from build123d import *

# Parameters (mm, degrees)
SKETCH2_R           = 31
SKETCH2_R_2         = 11.1
SKETCH2_R_3         = 3
BOSS_EXTRUDE1_DEPTH = 6
BOSS_EXTRUDE3_START = -3.9
SKETCH4_R           = 11.1
SKETCH4_R_2         = 5
BOSS_EXTRUDE3_DEPTH = 3.9
SKETCH5_R           = 2.3
CUT_EXTRUDE1_DEPTH  = 6
CIRPATTERN3_COUNT   = 4
CUT_EXTRUDE2_REACH  = 101.674
SKETCH12_R          = 3
CIRPATTERN4_COUNT   = 2
CIRPATTERN4_ANGLE   = 60
CIRPATTERN5_COUNT   = 4


# Read off the part's stored shape, not the designer's step: Revolve1
with BuildPart() as part:
    # Sketch2 → Boss-Extrude1 (new body)
    with BuildSketch(Plane(origin=(-62.154924708, 3.943558292, 10.8), x_dir=(1, 0, 0), z_dir=(0, 0, 1))):
        Circle(SKETCH2_R)
        Circle(SKETCH2_R_2, mode=Mode.SUBTRACT)
        with Locations((-15.5, 15.5)):
            Circle(SKETCH2_R_3, mode=Mode.SUBTRACT)
        with Locations((15.5, 15.5)):
            Circle(SKETCH2_R_3, mode=Mode.SUBTRACT)
        with Locations((15.5, -15.5)):
            Circle(SKETCH2_R_3, mode=Mode.SUBTRACT)
        with Locations((-15.5, -15.5)):
            Circle(SKETCH2_R_3, mode=Mode.SUBTRACT)
    extrude(amount=BOSS_EXTRUDE1_DEPTH)

    # Sketch4 → Boss-Extrude3 (add)
    with BuildSketch(Plane(origin=(-62.154924708, 3.943558292, 16.8), x_dir=(1, 0, 0), z_dir=(0, 0, 1)).offset(BOSS_EXTRUDE3_START)):
        Circle(SKETCH4_R)
        Circle(SKETCH4_R_2, mode=Mode.SUBTRACT)
    extrude(amount=BOSS_EXTRUDE3_DEPTH)

    # Sketch5 → Cut-Extrude1 (cut)
    with BuildSketch(Plane.XY.offset(16.8)):
        with Locations((-46.154924708, 3.943558292)):
            Circle(SKETCH5_R)
        with Locations((-54.154924708, -9.912848169)):
            Circle(SKETCH5_R)
        with Locations((-70.154924708, -9.912848169)):
            Circle(SKETCH5_R)
        with Locations((-78.154924708, 3.943558292)):
            Circle(SKETCH5_R)
        with Locations((-70.154924708, 17.799964752)):
            Circle(SKETCH5_R)
        with Locations((-54.154924708, 17.799964752)):
            Circle(SKETCH5_R)
    extrude(amount=-CUT_EXTRUDE1_DEPTH, mode=Mode.SUBTRACT)

    # Revolve1 outline → Revolve1 (revolve)
    with BuildSketch(Plane(origin=(-77.654924708, 19.443558292, 0), x_dir=(1, 0, 0), z_dir=(0, -1, 0))):
        Polygon((1.7, 13.915), (1.7, 10.8), (3, 10.8), (3, 15.215), align=None)
    revolve1 = revolve(axis=Axis((-77.654924708, 19.443558292, 0), (0, 0, 1)))

    # CirPattern3: Revolve1 ×4 about axis
    cirpattern3_axis = Axis((-62.154924708, 3.943558292, 0), (0, 0, 1))
    for i in range(1, CIRPATTERN3_COUNT):
        add(revolve1.rotate(cirpattern3_axis, i * 360 / CIRPATTERN3_COUNT))

    # Sketch12 → Cut-Extrude2 (cut, up to next)
    with BuildSketch(Plane(origin=(0, 0, 10.8), x_dir=(-1, 0, 0), z_dir=(0, 0, -1)), mode=Mode.PRIVATE) as cut_extrude2_sk1:
        with Locations((69.013629403, -21.653476105)):
            Circle(SKETCH12_R)
    cut_extrude2_tool1 = extrude(cut_extrude2_sk1.sketch, amount=-CUT_EXTRUDE2_REACH, mode=Mode.PRIVATE) & part.part
    # Sketch12 → Cut-Extrude2 (cut, up to next)
    with BuildSketch(Plane(origin=(0, 0, 10.8), x_dir=(-1, 0, 0), z_dir=(0, 0, -1)), mode=Mode.PRIVATE) as cut_extrude2_sk2:
        with Locations(Location((55.296220013, -21.653476105, 0), (0, 0, 180))):
            Circle(SKETCH12_R)
    cut_extrude2_tool2 = extrude(cut_extrude2_sk2.sketch, amount=-CUT_EXTRUDE2_REACH, mode=Mode.PRIVATE) & part.part
    # Sketch12 → Cut-Extrude2 (cut, up to next)
    with BuildSketch(Plane(origin=(0, 0, 10.8), x_dir=(-1, 0, 0), z_dir=(0, 0, -1)), mode=Mode.PRIVATE) as cut_extrude2_sk3:
        with Locations(Location((36.557890311, 10.802262987, 0), (0, 0, 180))):
            Circle(SKETCH12_R)
    cut_extrude2_tool3 = extrude(cut_extrude2_sk3.sketch, amount=-CUT_EXTRUDE2_REACH, mode=Mode.PRIVATE) & part.part
    # Sketch12 → Cut-Extrude2 (cut, up to next)
    with BuildSketch(Plane(origin=(0, 0, 10.8), x_dir=(-1, 0, 0), z_dir=(0, 0, -1)), mode=Mode.PRIVATE) as cut_extrude2_sk4:
        with Locations((36.557890311, -2.915146404)):
            Circle(SKETCH12_R)
    cut_extrude2_tool4 = extrude(cut_extrude2_sk4.sketch, amount=-CUT_EXTRUDE2_REACH, mode=Mode.PRIVATE) & part.part
    # Sketch12 → Cut-Extrude2 (cut, up to next)
    with BuildSketch(Plane(origin=(0, 0, 10.8), x_dir=(-1, 0, 0), z_dir=(0, 0, -1)), mode=Mode.PRIVATE) as cut_extrude2_sk5:
        with Locations(Location((69.013629403, 29.540592688, 0), (0, 0, 180))):
            Circle(SKETCH12_R)
    cut_extrude2_tool5 = extrude(cut_extrude2_sk5.sketch, amount=-CUT_EXTRUDE2_REACH, mode=Mode.PRIVATE) & part.part
    # Sketch12 → Cut-Extrude2 (cut, up to next)
    with BuildSketch(Plane(origin=(0, 0, 10.8), x_dir=(-1, 0, 0), z_dir=(0, 0, -1)), mode=Mode.PRIVATE) as cut_extrude2_sk6:
        with Locations((55.296220013, 29.540592688)):
            Circle(SKETCH12_R)
    cut_extrude2_tool6 = extrude(cut_extrude2_sk6.sketch, amount=-CUT_EXTRUDE2_REACH, mode=Mode.PRIVATE) & part.part
    # Sketch12 → Cut-Extrude2 (cut, up to next)
    with BuildSketch(Plane(origin=(0, 0, 10.8), x_dir=(-1, 0, 0), z_dir=(0, 0, -1)), mode=Mode.PRIVATE) as cut_extrude2_sk7:
        with Locations(Location((87.751959105, -2.915146404, 0), (0, 0, 180))):
            Circle(SKETCH12_R)
    cut_extrude2_tool7 = extrude(cut_extrude2_sk7.sketch, amount=-CUT_EXTRUDE2_REACH, mode=Mode.PRIVATE) & part.part
    # Sketch12 → Cut-Extrude2 (cut, up to next)
    with BuildSketch(Plane(origin=(0, 0, 10.8), x_dir=(-1, 0, 0), z_dir=(0, 0, -1)), mode=Mode.PRIVATE) as cut_extrude2_sk8:
        with Locations((87.751959105, 10.802262987)):
            Circle(SKETCH12_R)
    cut_extrude2_tool8 = extrude(cut_extrude2_sk8.sketch, amount=-CUT_EXTRUDE2_REACH, mode=Mode.PRIVATE) & part.part
    add(cut_extrude2_tool1.solids().sort_by_distance((-69.013629, -21.653476, 10.8))[0], mode=Mode.SUBTRACT)
    add(cut_extrude2_tool2.solids().sort_by_distance((-55.29622, -21.653476, 10.8))[0], mode=Mode.SUBTRACT)
    add(cut_extrude2_tool3.solids().sort_by_distance((-36.55789, 10.802263, 10.8))[0], mode=Mode.SUBTRACT)
    add(cut_extrude2_tool4.solids().sort_by_distance((-36.55789, -2.915146, 10.8))[0], mode=Mode.SUBTRACT)
    add(cut_extrude2_tool5.solids().sort_by_distance((-69.013629, 29.540593, 10.8))[0], mode=Mode.SUBTRACT)
    add(cut_extrude2_tool6.solids().sort_by_distance((-55.29622, 29.540593, 10.8))[0], mode=Mode.SUBTRACT)
    add(cut_extrude2_tool7.solids().sort_by_distance((-87.751959, -2.915146, 10.8))[0], mode=Mode.SUBTRACT)
    add(cut_extrude2_tool8.solids().sort_by_distance((-87.751959, 10.802263, 10.8))[0], mode=Mode.SUBTRACT)

    # Sketch18 → Revolve2 (revolve)
    with BuildSketch(Plane(origin=(-5.149480043, 19.218121154, 0), x_dir=(-0.9659258262890653, -0.25881904510253195, 0), z_dir=(0.25881904510253195, -0.9659258262890653, 0)), mode=Mode.PRIVATE) as revolve2_sk:
        Polygon((82.516379015, -10.8), (82.516379015, -15.215), (83.816379015, -13.915), (83.816379015, -10.8), align=None)
    revolve2 = revolve(revolve2_sk.sketch.rotate(Axis((-87.751959105, -2.915146404, 16.8), (0, 0, -1)), 15), axis=Axis((-87.751959105, -2.915146404, 16.8), (0, 0, -1)))

    # CirPattern4: Revolve2 ×2 about axis
    cirpattern4_axis = Axis((-62.154924708, 3.943558292, 0), (0, 0, 1))
    for i in range(1, CIRPATTERN4_COUNT):
        add(revolve2.rotate(cirpattern4_axis, i * CIRPATTERN4_ANGLE / (CIRPATTERN4_COUNT - 1)))

    # CirPattern5: Revolve2 ×4 about axis
    cirpattern5_axis = Axis((-62.154924708, 3.943558292, 0), (0, 0, -1))
    for i in range(1, CIRPATTERN5_COUNT):
        add(revolve2.rotate(cirpattern5_axis, i * 360 / CIRPATTERN5_COUNT))

    # CirPattern5 copy 1 sketch → CirPattern5 copy 1 (revolve)
    with BuildSketch(Plane(origin=(-5.149480043, -11.33100457, 0), x_dir=(-0.965925826289072, 0.2588190451025073, 0), z_dir=(-0.2588190451025073, -0.965925826289072, 0))):
        Polygon((82.516379015, -10.8), (82.516379015, -15.215), (83.816379015, -13.915), (83.816379015, -10.8), align=None)
    revolve(axis=Axis((-87.751959105, 10.802262987, 16.8), (0, 0, -1)))

    # CirPattern5 copy 2 sketch → CirPattern5 copy 2 (revolve)
    with BuildSketch(Plane(origin=(-77.42948757, -53.061886373, 0), x_dir=(0.2588190451025072, 0.965925826289072, 0), z_dir=(-0.965925826289072, 0.2588190451025072, 0))):
        Polygon((82.516379015, -10.8), (82.516379015, -15.215), (83.816379015, -13.915), (83.816379015, -10.8), align=None)
    revolve(axis=Axis((-55.296220013, 29.540592689, 16.8), (0, 0, -1)))

    # CirPattern5 copy 3 sketch → CirPattern5 copy 3 (revolve)
    with BuildSketch(Plane(origin=(-119.160369373, 19.218121154, 0), x_dir=(0.965925826289072, -0.25881904510250714, 0), z_dir=(0.25881904510250714, 0.965925826289072, 0))):
        Polygon((82.516379015, -10.8), (82.516379015, -15.215), (83.816379015, -13.915), (83.816379015, -10.8), align=None)
    revolve(axis=Axis((-36.557890311, -2.915146403, 16.8), (0, 0, -1)))


solid = part.part
CAD build for the part. Positions are in the model's coordinates, mm. A direction names the side the tool comes from. Coordinates: 2 decimals unless noted, no trailing zeros. Loops run counter-clockwise (first coordinate to the right, second up) from the corner with the lowest first, then second, coordinate; pieces in that order, holes last. Notation, with made-up numbers: (38.25, 47) - (96.25, 47) arc R33 ccw to (96.25, 84) - close; hole circle Ø8 at (-37.75, 43). An arc over 180 degrees is marked (long way). Write item = value, one per line. Start each with the question number.
Q1. Cut at B-B, the plane y = 23.5. List the corners of the cut face in (x, z).
Q2. Drill centre lines: L1, parallel to Y at x = -47, z = 13.2; L2, parallel to X at y = 10.5, z = 13.05; L3, parallel to Y at x = -56, z = 11.8. Where is each one in solid material? Low to high.
Q3. Pull direction Y, two halves, no side cores. Call faces 4 (the cylindrical face through (-32.6, 13.3, 13.8)), 5 (the cylindrical face through (-48.225, -10.905, 12.336)), 6 (the flat face through (-56, 4, 16.8)): pulls with the +Y half, pulls with the -Y half, needs draft (parallel to the pull), parting line crosses it, or undercut.
Q4. Flat gauge pins, fed straight in: pin 1 Ø1.5 at (x, z) = (-68, 13.5) entering from -Y; pin 2 Ø1.5 at (x, z) = (-42.5, 15.5) entering from +Y; pin 3 Ø1.5 at (x, z) = (-80, 16) entering from -Y. Where does each tip first touch, or does it go through?
Q5. Which spindle directions (+Z, -Z, +X, -X, +Y, -Y) get a long thin tool onto all of the face, cutting with end or side? Do faces 1 (the cylindrical face through (-33.787, 11.951, 15.996)), 2 (the cylindrical face through (-73.244, 4.432, 11.835)), 3 (the cylindrical face through (-34.86, 10.88, 12.34)). Say none if no direction does.
Q6. Cut at A-A, the plane z = 12. Give the number of separate pieces and of enclosed holes in the cut face, then the cut area to 3 significant figures.
Computed:
q1.outline = (-86.21, 10.8) - (-38.1, 10.8) - (-38.1, 16.8) - (-86.21, 16.8) - close
q2.L1 = -23.1 to -13.22, -9.89 to 1.8, 6.08 to 17.78, 21.11 to 30.99
q2.L2 = -92.45 to -89.42, -86.08 to -38.23, -34.88 to -31.86
q2.L3 = -26.44 to -23.2, -20.11 to -11.29, -8.54 to -5.29, 13.18 to 16.43, 19.17 to 27.99, 31.09 to 34.33
q3.face_4 = parting line crosses it
q3.face_5 = undercut
q3.face_6 = needs draft
q4.pin_1 = -26.63
q4.pin_2 = 28.51
q4.pin_3 = -21.92
q5.face_1 = +Z
q5.face_2 = -Z
q5.face_3 = +Z, -Z
q6.separate_pieces = 1
q6.enclosed_holes = 19
q6.area = 2,420 mm²
